from build123d import *

# Parameters (mm, degrees)
SKETCH_1_R          = 2.5
EXTRUDE_1_DEPTH     = 71
CHAMFER_1_SIZE      = 0.5
CUT_EXTRUDE_START   = -15
CUT_EXTRUDE_2_DEPTH = 15


with BuildPart() as part:
    # Эскиз1 → Бобышка-Вытянуть1 (new body)
    with BuildSketch(Plane(origin=(0, 0, 0), x_dir=(1, 0, 0), z_dir=(0, 1, 0))):
        with Locations(Location((0, 0, 0), (0, 0, 270))):
            Circle(SKETCH_1_R)
    extrude(amount=EXTRUDE_1_DEPTH)

    # Фаска1
    chamfer_1_edges = [part.edges().sort_by_distance(p)[0] for p in [
        (0, 0, -2.5),
        (0, 71, -2.5),
    ]]
    chamfer(chamfer_1_edges, length=CHAMFER_1_SIZE)

    # Вырез-Вытянуть1 cone 1 section (through the dimple's axis) → Вырез-Вытянуть1 (revolve, cut)
    with BuildSketch(Plane(origin=(0, 71, 0), x_dir=(0, 0, 1), z_dir=(1, 0, 0))):
        Polygon((0, 0), (0.368933835, 0), (0, 0.913143285), align=None)
    revolve(axis=Axis((0, 71, 0), (0, -1, 0)), mode=Mode.SUBTRACT)

    # Эскиз3 → Вырез-Вытянуть2 (cut)
    with BuildSketch(Plane(origin=(0, 71, 0), x_dir=(1, 0, 0), z_dir=(0, 1, 0)).offset(CUT_EXTRUDE_START)):
        with BuildLine():
            Line((-1.5, 2), (1.5, 2))
            ThreePointArc((1.5, 2), (0, 2.5), (-1.5, 2))
        make_face()
    extrude(amount=CUT_EXTRUDE_2_DEPTH, mode=Mode.SUBTRACT)


solid = part.part
Build history of the part. All positions in model axes, mm. A direction names the side the tool comes from. Coordinates: 2 decimals unless noted, no trailing zeros. Write each loop counter-clockwise with the first axis right and the second up, starting at its lowest first coordinate (ties: lowest second). Pieces come first, ordered by that corner, then holes.
(1) Cut at A-A on y = 67.5. List the corners of the cut face in (x, z).
(2) 3-axis set-ups, long thin cutter, end or side, ignore diameter. For faces 1 (the flat face through (0, 63, -2)), 2 (the flat face through (0, 0, 0)): which of +Z, -Z, +X, -X, +Y, -Y reach the whole face in a straight line?
(3) Drill centre lines: line 1 (Z direction, x = -0.15, y = 63.5); line 2 (Z direction, x = -1.5, y = 64); line 3 (X direction, y = 36, z = 1.7). Where is each one in solid material? Low to high.
(4) Cut at B-B on y = 23. List the corners of the cut face in (x, z), and give its area (3 significant figures).
(5) Pin check, flat tips, straight feed: pin 1 Ø2 at (y, z) = (30.5, -1.5) entering from +X; pin 2 Ø1.5 at (x, y) = (0.5, 61.5) entering from -Z. Stop position of each tip, or through.
Working result:
1. outline: (-1.5, -2) - (1.5, -2) arc R2.5 ccw (long way) to start
2. face 1: -Z, +X, -X, +Y
2. face 2: +Z, -Z, +X, -X, -Y
3. line 1: z = -2 to 2.5
3. line 2: z = -2 to 2
3. line 3: x = -1.83 to 1.83
4. outline: circle Ø5 at (0, 0)
4. area: 19.6 mm2
5. pin 1: stops at x = 2.45
5. pin 2: stops at z = -2
